The listing builds one solid part. Answer for the finished solid, in the listing's coordinates (mm). Face numbers are marked on the shaded views. A direction names the side the tool comes from. Round coordinates to 2 decimals unless told otherwise and drop trailing zeros. Loops run counter-clockwise (first coordinate to the right, second up) from the corner with the lowest first, then second, coordinate; pieces in that order, holes last. Notation, with made-up numbers: (21.5, 64.5) -> (64.5, 64.5) arc R22 ccw to (64.5, 84.5) -> close; hole circle Ø8 at (-12, -32). An arc over 180 degrees is marked (long way). Answer in a Markdown table with one row per item. Add a question column.
Autodesk Inventor part; units mm, degrees
ref_plane "YZ Plane" through (0, 0, 0) normal (1, 0, 0) x (0, 1, 0)
ref_plane "XZ Plane" through (0, 0, 0) normal (0, 1, 0) x (-1, 0, 0)
ref_plane "XY Plane" through (0, 0, 0) normal (0, 0, 1) x (1, 0, 0)
sketch "Skizze1" plane through (0, 0, 0) normal (0, 0, 1) x (1, 0, 0)
  line L0 (-17.5, 7.5) -> (-17.5, 6.5)
  line L1 (-17.5, 6.5) -> (-13.5, 6.5)
  line L2 (-13.5, 6.5) -> (-13.5, 0)
  line L3 (-13.5, 0) -> (13.5, 0)
  line L4 (13.5, 0) -> (13.5, 6.5)
  line L5 (13.5, 6.5) -> (17.5, 6.5)
  line L6 (17.5, 6.5) -> (17.5, 7.5)
  line L7 (17.5, 7.5) -> (11, 7.5)
  line L8 (-11, 7.5) -> (-17.5, 7.5)
  line L9 (0, -1.5) -> (0, 9) construction
  line L10 (-11, 2.5) -> (11, 2.5)
  line L11 (-11, 7.5) -> (-11, 2.5)
  line L12 (11, 2.5) -> (11, 7.5)
  line L13 (-13.5, 0) -> (-17.5, 0)
  line L14 (-17.5, 0) -> (-17.5, 6.5)
  line L15 (-17.5, 6.5) -> (-13.5, 6.5)
  line L16 (-13.5, 6.5) -> (-13.5, 0)
  point P0 (0, 0)
  point P1 (0, 2.5)
  dimension "d0" = 1
  dimension "d1" = 35
  dimension "d2" = 27
  dimension "d3" = 7.5
  dimension "d6" = 4
  dimension "d7" = 2.5
  dimension "d8" = 2.5
extrude "Extrusion1" add sketch "Skizze1" along normal mid plane 18 contours L8 L11 L10 L12 L7 L6 L5 L4 L3 L2 L1 L0
extrude "Extrusion2" add sketch "Skizze1" along normal mid plane 11 contours L1 L2 L13 L14
sketch "Skizze2" plane through (-11, 2.5, 9) normal (0, 1, 0) x (1, 0, 0)
  line L0 (0, 18) -> (0, 0)
  line L1 (22, 0) -> (0, 0)
  line L2 (22, 18) -> (22, 0)
  line L3 (0, 18) -> (22, 18)
  line L4 (0, 9) -> (22, 9) construction
  line L5 (11, 0) -> (11, 18) construction
  point P0 (11, 9)
  point P1 (5.5, 9)
  point P2 (16.5, 9)
  dimension "d13" = 11
  dimension "d14" = 22
hole "Bohrung1" at (-5.5, 2.5, 0) at (5.5, 2.5, 0) direction (0, -1, 0) diameter 4.5 end through all
properties part number "Hutschiene"
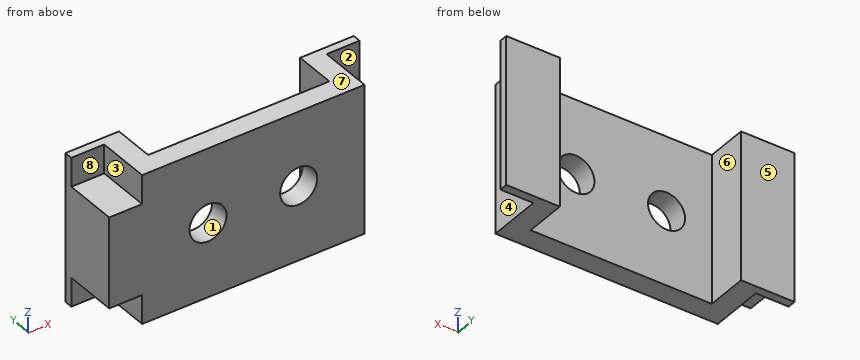
Item 1: For the marked faces 4, 5, 6, 7 and 8, determine the directions among +Z, -Z, +X, -X, +Y, -Y from which every point of the face is accessible in a straight line to the end or side of a thin tool.
Item 2: Section D-D, the plane z = -4.5 is taken. Write down the section's boundary in (x, y).
Item 3: Flat-ended cylindrical pins translate along their axes: P1, Ø1.5, axis at y = 4.5, z = 4.5, coming from the +X side; P2, Ø1, axis at y = 3, z = -7, coming from the -X side; P3, Ø10, axis at x = -3.5, z = 0.5, coming from the +Y side. Find the tip coordinate at first contact, or state that the pin passes through.
Item 4: Section B-B, the plane z = 0 is taken. Write down the section's boundary in (x, y).
Item 5: The mould has two halves that part along X. Classify the marked faces 1, 2 and 3: +X half, -X half, draft (parallel to the pull), parting line (faces both ways), or undercut.
Item 6: Consider L1, parallel to X at y = 1.65, z = 0; L2, parallel to Z at x = -5.5, y = 0.7; L3, parallel to X at y = 3.75, z = -8. Determine where each line is inside the solid, lowest interval first. Write a range as from..to.
Item 7: Section A-A, the plane x = 5.5 is taken. Write down the section's boundary in (y, z).
Item 8: Section C-C, the plane y = 1 is taken. Write down the section's boundary in (x, z), and give its area (3 significant figures).
Here are the results:
| question | item | result |
|---|---|---|
| 1 | face 4 | +Z, -Z, +X, -Y |
| 1 | face 5 | +Z, -Z, +X, -X, +Y |
| 1 | face 6 | +Z, -Z, +Y |
| 1 | face 7 | +Z, +X, -X, +Y, -Y |
| 1 | face 8 | +Z, -X, -Y |
| 2 | outline | (-17.5, 0) -> (13.5, 0) -> (13.5, 6.5) -> (17.5, 6.5) -> (17.5, 7.5) -> (11, 7.5) -> (11, 2.5) -> (-11, 2.5) -> (-11, 7.5) -> (-17.5, 7.5) -> close |
| 3 | P1 | stops at x = 13.5 |
| 3 | P2 | stops at x = -13.5 |
| 3 | P3 | stops at y = 2.5 |
| 4 | outline | (-17.5, 0) -> (-7.75, 0) -> (-7.75, 2.5) -> (-11, 2.5) -> (-11, 7.5) -> (-17.5, 7.5) -> close; (-3.25, 0) -> (3.25, 0) -> (3.25, 2.5) -> (-3.25, 2.5) -> close; (7.75, 0) -> (13.5, 0) -> (13.5, 6.5) -> (17.5, 6.5) -> (17.5, 7.5) -> (11, 7.5) -> (11, 2.5) -> (7.75, 2.5) -> close |
| 5 | face 1 | undercut |
| 5 | face 2 | draft |
| 5 | face 3 | -X half |
| 6 | L1 | x = -17.5..-7.75, -3.25..3.25, 7.75..13.5 |
| 6 | L2 | z = -9..-2.25, 2.25..9 |
| 6 | L3 | x = -13.5..-11, 11..13.5 |
| 7 | outline | (0, -9) -> (2.5, -9) -> (2.5, -2.25) -> (0, -2.25) -> close; (0, 2.25) -> (2.5, 2.25) -> (2.5, 9) -> (0, 9) -> close |
| 8 | outline | (-17.5, -5.5) -> (-13.5, -5.5) -> (-13.5, -9) -> (13.5, -9) -> (13.5, 9) -> (-13.5, 9) -> (-13.5, 5.5) -> (-17.5, 5.5) -> close; hole circle Ø4.5 at (-5.5, 0); hole circle Ø4.5 at (5.5, 0) |
| 8 | area | 498 mm² |
